Autodesk Fusion 360 part; units mm, degrees
sketch "Sketch1" plane through (0, 0, 0) normal (0, 0, 1) x (1, 0, 0)
  line L0 (-64, 66.5) -> (64, 66.5)
  line L1 (66.5, 64) -> (66.5, -64)
  line L2 (64, -66.5) -> (-36.5, -66.5)
  line L3 (-66.5, -36.5) -> (-66.5, 64)
  line L4 (-36.5, -66.5) -> (-66.5, -36.5)
  arc A0 (-64, 66.5) -> (-66.5, 64) centre (-64, 64) ccw
  arc A1 (66.5, 64) -> (64, 66.5) centre (64, 64) ccw
  arc A2 (64, -66.5) -> (66.5, -64) centre (64, -64) ccw
extrude "Extrude1" add sketch "Sketch1" along normal blind 5
sketch "Sketch2" plane through (0, 0, 5) normal (0, 0, 1) x (-1, 0, 0)
  line L0 (36.5, 66.5) -> (-64, 66.5)
  arc A0 (-64, 66.5) -> (-66.5, 64) centre (-64, 64) ccw
  line L1 (-66.5, 64) -> (-66.5, -64)
  arc A1 (-66.5, -64) -> (-64, -66.5) centre (-64, -64) ccw
  line L2 (-64, -66.5) -> (64, -66.5)
  arc A2 (64, -66.5) -> (66.5, -64) centre (64, -64) ccw
  line L3 (66.5, -64) -> (66.5, 36.5)
  line L4 (66.5, 36.5) -> (36.5, 66.5)
  circle A3 centre (0, 0) radius 20
  circle A4 centre (0, 0) radius 16.5
  line L5 (-56.5, -66.5) -> (56.5, -66.5)
  line L6 (56.5, -66.5) -> (56.5, -50.5727)
  line L7 (49, -43.0727) -> (-49, -43.0727)
  line L8 (-56.5, -50.5727) -> (-56.5, -66.5)
  arc A5 (56.5, -50.5727) -> (49, -43.0727) centre (49, -50.5727) ccw
  arc A6 (-49, -43.0727) -> (-56.5, -50.5727) centre (-49, -50.5727) ccw
Geometry check sheet. Reference: the model listing, model coordinates, mm. Round coordinates to 2 decimals unless told otherwise and drop trailing zeros. Write each loop counter-clockwise with the first axis right and the second up, starting at its lowest first coordinate (ties: lowest second). Pieces come first, ordered by that corner, then holes.
Item 1: Section check B-B (x = -49). Record the boundary of the cut face in (y, z).
Determined:
outline: (-54, 0) - (66.5, 0) - (66.5, 5) - (-54, 5) - close
Item 2: Material ranges on line 1 along X through (y, z) = (-46.5, 2.4); line 2 along Y through (x, z) = (-51, 2.4); line 3 along X through (y, z) = (-45, 4.8), recorded low to high.
Determined:
line 1: x = -56.5 to 66.5
line 2: y = -52 to 66.5
line 3: x = -58 to 66.5
Item 3: Go/stop test with a flat-tipped pin: pin 1 Ø1 at (x, z) = (-48.5, 3) entering from -Y. Record where the tip stops, or that it passes through.
Determined:
pin 1: stops at y = -55
Item 4: Section check A-A (z = 4.1). Record the boundary of the cut face in (x, y).
Determined:
outline: (-66.5, -36.5) - (-36.5, -66.5) - (64, -66.5) arc R2.5 ccw to (66.5, -64) - (66.5, 64) arc R2.5 ccw to (64, 66.5) - (-64, 66.5) arc R2.5 ccw to (-66.5, 64) - close
